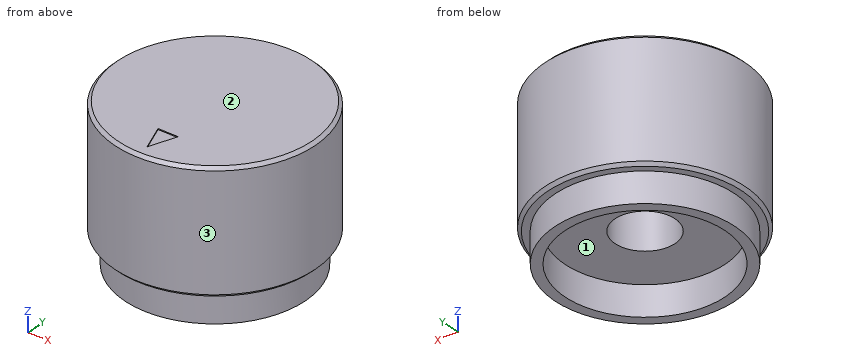
from build123d import *

# Parameters (mm, degrees)
SKETCH1_R           = 10
BOSS_EXTRUDE1_DEPTH = 12
SKETCH2_R           = 9
SKETCH2_R_2         = 8
BOSS_EXTRUDE2_DEPTH = 3
SKETCH3_R           = 3
CUT_EXTRUDE1_DEPTH  = 10
CHAMFER1_SIZE       = 0.3
CUT_EXTRUDE2_DEPTH  = 0.1


with BuildPart() as part:
    # Sketch1 → Boss-Extrude1 (new body)
    with BuildSketch(Plane(origin=(0, 0, 0), x_dir=(0, 1, 0), z_dir=(0, 0, 1))):
        with Locations(Location((0, 0, 0), (0, 0, 270))):
            Circle(SKETCH1_R)
    extrude(amount=BOSS_EXTRUDE1_DEPTH)

    # Sketch2 → Boss-Extrude2 (add)
    with BuildSketch(Plane(origin=(0, 0, 0), x_dir=(1, 0, 0), z_dir=(0, 0, -1))):
        Circle(SKETCH2_R)
        with Locations(Location((0, 0, 0), (0, 0, 180))):
            Circle(SKETCH2_R_2, mode=Mode.SUBTRACT)
    extrude(amount=BOSS_EXTRUDE2_DEPTH)

    # Sketch3 → Cut-Extrude1 (cut)
    with BuildSketch(Plane(origin=(0, 0, 0), x_dir=(1, 0, 0), z_dir=(0, 0, -1))):
        with Locations(Location((0, 0, 0), (0, 0, 180))):
            Circle(SKETCH3_R)
    extrude(amount=-CUT_EXTRUDE1_DEPTH, mode=Mode.SUBTRACT)

    # Chamfer1
    chamfer1_edges = [part.edges().sort_by_distance(p)[0] for p in [
        (-10, 0, 0),
        (-10, 0, 12),
    ]]
    chamfer(chamfer1_edges, length=CHAMFER1_SIZE)

    # Sketch4 → Cut-Extrude2 (cut)
    with BuildSketch(Plane.XY.offset(12)):
        Polygon((-1, -6), (1, -6), (0, -8.7), align=None)
    extrude(amount=-CUT_EXTRUDE2_DEPTH, mode=Mode.SUBTRACT)


solid = part.part
Could you check a few things on this model? Use its own coordinates, in mm. Face numbers are marked on the shaded views. Round coordinates to 2 decimals unless told otherwise and drop trailing zeros. Order: outer loops, then holes, each group sorted by start corner. A loop starts at its lowest first (then second) coordinate and runs counter-clockwise, first axis right, second up.
Q1. Please list where these lines run through material, in increasing order: probe 1 along Y at (x, z) = (0, 8); probe 2 along Y at (x, z) = (0, -1.85); probe 3 along Z at (x, y) = (1.25, -2.25).
Geometry says:
probe 1: y = -10 to -3, 3 to 10
probe 2: y = -9 to -8, 8 to 9
probe 3: z = 10 to 12
Q2. Imagine slicing it at B-B, the plane y = 0. List the corners of the cut face in (x, z) for me.
Geometry says:
outline: (-10, 0.3) - (-9.7, 0) - (-9, 0) - (-9, -3) - (-8, -3) - (-8, 0) - (-3, 0) - (-3, 10) - (3, 10) - (3, 0) - (8, 0) - (8, -3) - (9, -3) - (9, 0) - (9.7, 0) - (10, 0.3) - (10, 11.7) - (9.7, 12) - (-9.7, 12) - (-10, 11.7) - close
Q3. Thinking about a two-plate mould opening in X: for the marked faces 1, 2 and 3, which applies, released by +X, released by -X, zero draft, split by the parting line, or undercut?
Geometry says:
face 1: undercut
face 2: zero draft
face 3: split by the parting line
Q4. Imagine slicing it at A-A, the plane z = 6.25. List the corners of the cut face in (x, y) for me.
Geometry says:
outline: circle Ø20 at (0, 0); hole circle Ø6 at (0, 0)
Q5. I'm going to push flat-ended pins straight in: P1, Ø3, axis at x = 1.5, y = 6, coming from the -Z side; P2, Ø1.8, axis at x = -1, y = 0.5, coming from the -Z side; P3, Ø1, axis at y = -4.5, z = 0, coming from the -X side. Where does each tip first touch, or does it pass through?
Geometry says:
P1: stops at z = 0
P2: stops at z = 10
P3: stops at x = -9.12
